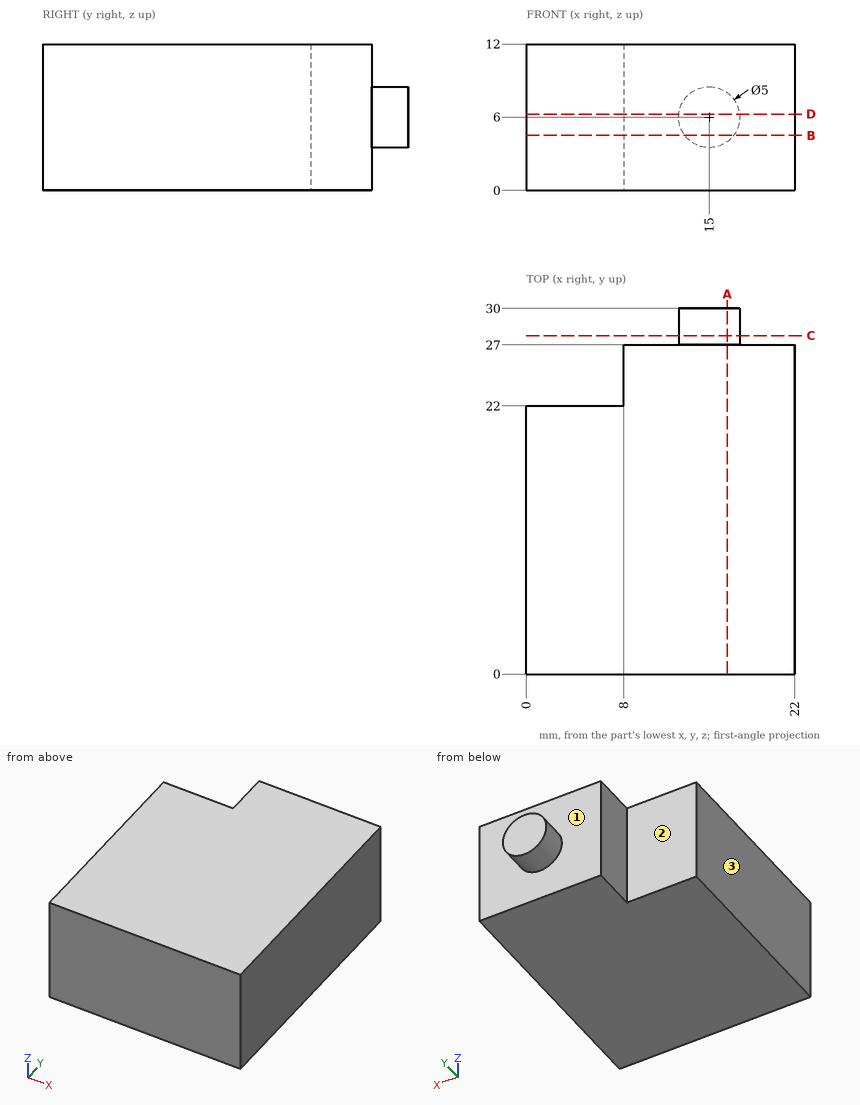
Job drawing, mm, ordinate dimensions from the low corner. One solid piece. A direction names the side the tool comes from. Give positions to 0.01 mm unless a question says otherwise; leave off trailing zeros. Loops run counter-clockwise (first coordinate to the right, second up) from the corner with the lowest first, then second, coordinate; pieces in that order, holes last. Notation, with made-up numbers: M 43.5,-23 L 91.5,-23 A25 cw 91.5,14 Z; hole C 43.5,31 d3. An arc over 180 degrees is marked long. Answer in a Markdown table with one row per item. Add a question column.
Item 1: Band-saw the part on C-C on y = 27.75. Give the cut face in (x, z), then the cut area to 3 significant figures.
Item 2: Probe probe 1 along Y at (x, z) = (7.75, 6.25); probe 2 along Y at (x, z) = (13, 10.5); probe 3 along X at (y, z) = (26, 4.75). List the from-to ranges inside material, lowest first.
Item 3: Band-saw the part on D-D on z = 6.25. Give the cut face in (x, y), then the cut area to 3 significant figures.
Item 4: Tool access for the marked faces 1, 2 and 3: list every direction of +Z, -Z, +X, -X, +Y, -Y with a clear straight run to the whole face (end or side of a thin tool).
Item 5: Drop flat-ended pins along their axis: P1, Ø4, axis at x = 3, z = 6.5, coming from the +Y side; P2, Ø3, axis at x = 8.5, z = 3, coming from the +Y side. Give the stop position or say it passes through.
Item 6: Band-saw the part on B-B on z = 4.5. Give the cut face in (x, y), then the cut area to 3 significant figures.
Item 7: Band-saw the part on A-A on x = 16.5. Give the cut face in (y, z), then the cut area to 3 significant figures.
Reply:
| question | item | result |
|---|---|---|
| 1 | outline | C 15,6 d5 |
| 1 | area | 19.6 mm^2 |
| 2 | probe 1 | y = 0 to 22 |
| 2 | probe 2 | y = 0 to 27 |
| 2 | probe 3 | x = 8 to 22 |
| 3 | outline | M 0,0 L 22,0 L 22,27 L 17.49,27 L 17.49,30 L 12.51,30 L 12.51,27 L 8,27 L 8,22 L 0,22 Z |
| 3 | area | 569 mm^2 |
| 4 | face 1 | +Y |
| 4 | face 2 | +Z, -Z, -X, +Y |
| 4 | face 3 | +Z, -Z, -X, +Y, -Y |
| 5 | P1 | stops at y = 22 |
| 5 | P2 | stops at y = 27 |
| 6 | outline | M 0,0 L 22,0 L 22,27 L 17,27 L 17,30 L 13,30 L 13,27 L 8,27 L 8,22 L 0,22 Z |
| 6 | area | 566 mm^2 |
| 7 | outline | M 0,0 L 27,0 L 27,4 L 30,4 L 30,8 L 27,8 L 27,12 L 0,12 Z |
| 7 | area | 336 mm^2 |
